Check sheet for the modelled part. Datum: model origin and axes. Units: mm. Coordinates: 2 decimals unless noted, no trailing zeros. Write each loop counter-clockwise with the first axis right and the second up, starting at its lowest first coordinate (ties: lowest second). Pieces come first, ordered by that corner, then holes. Notation, with made-up numbers: (60.25, -18.5) -> (79.25, -18.5) arc R25 cw to (79.25, -5.5) -> close; hole circle Ø9 at (2.5, 73). An arc over 180 degrees is marked (long way). One line per item, written item: value. Start each with the question number.
1) Sectioned sample at B-B on x = -95.25. Enter the section's corners in (y, z), plus the area to 3 significant figures.
2) Sectioned sample at A-A on y = 0. Enter the section's corners in (x, z) (3 decimals).
3) Scan lines: line 1 along X through (y, z) = (-68, 1.75); line 2 along Y through (x, z) = (95.25, 2.25); line 3 along X through (y, z) = (12.7, 1.75). Record each from-to range of solid material in increasing order. Write a range as [from, to].
4) Gauge pin test, flat ends, axial feed: P1, Ø1, axis at y = -41.5, z = 1, coming from the +X side; P2, Ø5.5, axis at x = 95.25, y = 12.7, coming from the +Z side; P3, Ø1.5, axis at x = 51.5, z = 2, coming from the -Y side; P4, Ø1, axis at y = 11.5, z = 4, coming from the -X side. Record the tip position at first contact, or that the pin passes through.
5) Sectioned sample at D-D on x = 27. Enter the section's corners in (y, z), plus the area to 3 significant figures.
6) Sectioned sample at C-C on z = 3.25. Give the number of separate pieces and of enclosed holes in the cut face, plus the area to 3 significant figures.
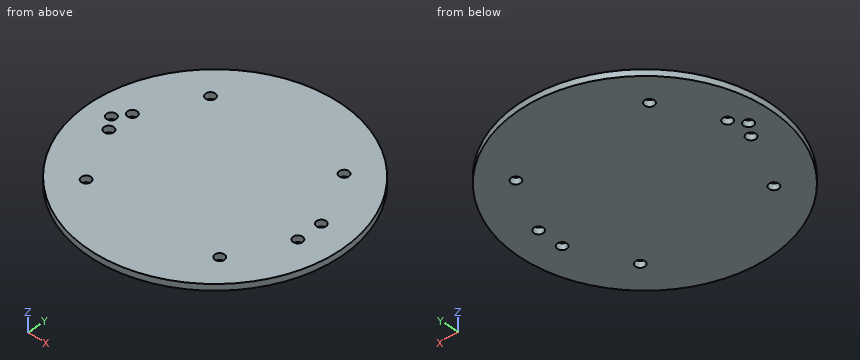
```python
from build123d import *

# Parameters (mm, degrees)
SKETCH1_R               = 127
BOSS_EXTRUDE1_DEPTH     = 6.35
CUT_EXTRUDE1_DEPTH      = 180.717340566
CUT_EXTRUDE1_DEPTH_BACK = 180.717340566
SKETCH2_R               = 4.7625
CUT_EXTRUDE2_DEPTH      = 180.717340566
CUT_EXTRUDE2_DEPTH_BACK = 180.717340566
SKETCH3_R               = 4.7625
CUT_EXTRUDE4_DEPTH      = 180.717340566
CUT_EXTRUDE4_DEPTH_BACK = 180.717340566
SKETCH4_R               = 4.7625


with BuildPart() as part:
    # Sketch1 → Boss-Extrude1 (new body)
    with BuildSketch(Plane.XY):
        Circle(SKETCH1_R)
    extrude(amount=BOSS_EXTRUDE1_DEPTH)

    # Sketch2 → Cut-Extrude1 (cut, two sides: drawn at the far end of the back side and taken through both)
    with BuildSketch(Plane.XY.offset(6.35).offset(-CUT_EXTRUDE1_DEPTH_BACK)):
        with Locations((-67.351920908, 67.351920908)):
            Circle(SKETCH2_R)
        with Locations((-67.351920908, -67.351920908)):
            Circle(SKETCH2_R)
        with Locations((67.351920908, -67.351920908)):
            Circle(SKETCH2_R)
        with Locations((67.351920908, 67.351920908)):
            Circle(SKETCH2_R)
    extrude(amount=CUT_EXTRUDE1_DEPTH + CUT_EXTRUDE1_DEPTH_BACK, mode=Mode.SUBTRACT)

    # Sketch3 → Cut-Extrude2 (cut, two sides: drawn at the far end of the back side and taken through both)
    with BuildSketch(Plane.XY.offset(6.35).offset(-CUT_EXTRUDE2_DEPTH_BACK)):
        with Locations((-95.25, 12.7)):
            Circle(SKETCH3_R)
        with Locations((-95.25, -12.7)):
            Circle(SKETCH3_R)
        with Locations((95.25, -12.7)):
            Circle(SKETCH3_R)
        with Locations((95.25, 12.7)):
            Circle(SKETCH3_R)
    extrude(amount=CUT_EXTRUDE2_DEPTH + CUT_EXTRUDE2_DEPTH_BACK, mode=Mode.SUBTRACT)

    # Sketch4 → Cut-Extrude4 (cut, two sides: drawn at the far end of the back side and taken through both)
    with BuildSketch(Plane.XY.offset(6.35).offset(-CUT_EXTRUDE4_DEPTH_BACK)):
        with Locations((-104.537500094, 0)):
            Circle(SKETCH4_R)
    extrude(amount=CUT_EXTRUDE4_DEPTH + CUT_EXTRUDE4_DEPTH_BACK, mode=Mode.SUBTRACT)


solid = part.part
```
Answers:
1. outline: (-84, 0) -> (-17.46, 0) -> (-17.46, 6.35) -> (-84, 6.35) -> close; (-7.94, 0) -> (7.94, 0) -> (7.94, 6.35) -> (-7.94, 6.35) -> close; (17.46, 0) -> (84, 0) -> (84, 6.35) -> (17.46, 6.35) -> close
1. area: 946 mm2
2. outline: (-127, 0) -> (-109.3, 0) -> (-109.3, 6.35) -> (-127, 6.35) -> close; (-99.775, 0) -> (127, 0) -> (127, 6.35) -> (-99.775, 6.35) -> close
3. line 1: x = [-107.26, -72.07], [-62.63, 62.63], [72.07, 107.26]
3. line 2: y = [-84, -17.46], [-7.94, 7.94], [17.46, 84]
3. line 3: x = [-126.36, -100.01], [-90.49, 90.49], [100.01, 126.36]
4. P1: stops at x = 120.2
4. P2: passes through
4. P3: stops at y = -116.42
4. P4: stops at x = -126.52
5. outline: (-124.1, 0) -> (124.1, 0) -> (124.1, 6.35) -> (-124.1, 6.35) -> close
5. area: 1,580 mm2
6. separate pieces: 1
6. enclosed holes: 9
6. area: 50,000 mm2
